Work out the finished part from the listing and answer in its coordinate system (mm). A direction names the side the tool comes from. Coordinates: 2 decimals unless noted, no trailing zeros. Order: outer loops, then holes, each group sorted by start corner. A loop starts at its lowest first (then second) coordinate and runs counter-clockwise, first axis right, second up. Notation, with made-up numbers: M 29,9.25 L 40,9.25 A26 ccw 40,37.25 Z; hole C 35,24 d7. An arc over 180 degrees is marked long. Answer in a Markdown table with one row per item. Add a question column.
Item 1: Which of the six approach directions +Z, -Z, +X, -X, +Y, -Y give full straight-line access (tool end or side, diameter ignored) to faces 1 (the face through (8.098, 0.66, 14.985)), 2 (the face through (20, -6, -20))?
Item 2: The part is cut by section C-C (x = 14). Write down the section's boundary in (y, z).
Item 3: The mould has two halves that part along Y. Classify faces 3 (the face through (0, 0, 0)), 4 (the face through (8, -21, 28)), 5 (the face through (1, 0, 0)): released by +Y, released by -Y, zero draft, split by the parting line, or undercut.
Item 4: Flat-ended cylindrical pins translate along their axes: pin 1 Ø24 at (y, z) = (0, 0) entering from +X; pin 2 Ø1.5 at (x, z) = (11, 3.5) entering from +Y; pin 3 Ø1 at (x, z) = (5.5, 21.5) entering from -Y. Find the tip coordinate at first contact, or state that the pin passes through.
Item 5: Consider line 1 (Y direction, x = 8, z = 0); line 2 (Y direction, x = 13.25, z = 4.5); line 3 (Z direction, x = 14, y = 6). Determine where each line is inside the solid, lowest interval first. Write a range as from..to.
Item 6: The part is cut by section A-A (y = 0). Write down the section's boundary in (x, z), then the cut area to 3 significant figures.
from build123d import *

# Parameters (mm, degrees)
SKETCH1_R           = 35
BOSS_EXTRUDE1_DEPTH = 20
SKETCH2_R           = 15
CUT_EXTRUDE1_DEPTH  = 19
FILLET1_R           = 5
FILLET2_R           = 1


with BuildPart() as part:
    # Sketch1 → Boss-Extrude1 (new body)
    with BuildSketch(Plane(origin=(0, 0, 0), x_dir=(0, 0, -1), z_dir=(1, 0, 0))):
        Circle(SKETCH1_R)
    extrude(amount=BOSS_EXTRUDE1_DEPTH)

    # Sketch2 → Cut-Extrude1 (cut)
    with BuildSketch(Plane(origin=(20, 0, 0), x_dir=(0, 0, -1), z_dir=(1, 0, 0))):
        Circle(SKETCH2_R)
    extrude(amount=-CUT_EXTRUDE1_DEPTH, mode=Mode.SUBTRACT)

    # Fillet1
    fillet1_edges = [part.edges().sort_by_distance(p)[0] for p in [
        (20, 0, 35),
        (20, 0, 15),
    ]]
    fillet(fillet1_edges, radius=FILLET1_R)

    # Fillet2
    fillet2_edges = [part.edges().sort_by_distance(p)[0] for p in [
        (0, 0, 35),
    ]]
    fillet(fillet2_edges, radius=FILLET2_R)


solid = part.part
Reply:
| question | item | result |
|---|---|---|
| 1 | face 1 | +X |
| 1 | face 2 | +Z, -Z, +X, +Y, -Y |
| 2 | outline | C 0,0 d70; hole C 0,0 d30 |
| 3 | face 3 | zero draft |
| 3 | face 4 | split by the parting line |
| 3 | face 5 | undercut |
| 4 | pin 1 | stops at x = 1 |
| 4 | pin 2 | stops at y = 34.89 |
| 4 | pin 3 | stops at y = -28 |
| 5 | line 1 | y = -35..-15, 15..35 |
| 5 | line 2 | y = -34.71..-14.31, 14.31..34.71 |
| 5 | line 3 | z = -34.48..-13.75, 13.75..34.48 |
| 6 | outline | M 0,-34 A1 ccw 1,-35 L 15,-35 A5 ccw 20,-30 L 20,-20 A5 ccw 15,-15 L 1,-15 L 1,15 L 15,15 A5 ccw 20,20 L 20,30 A5 ccw 15,35 L 1,35 A1 ccw 0,34 Z |
| 6 | area | 808 mm2 |
